Geometry: final body of the model. Coordinates: model frame, mm. A direction names the side the tool comes from. Give positions to 0.01 mm unless a question says otherwise; leave off trailing zeros. Loops run counter-clockwise (first coordinate to the right, second up) from the corner with the lowest first, then second, coordinate; pieces in that order, holes last. Notation, with made-up numbers: M 88,-34.75 L 94,-34.75 A19 cw 94,-22.75 Z; hole C 80,-39 d10. An arc over 180 degrees is marked long. Put each result on its own line as item: value.
```python
from build123d import *

# Parameters (mm, degrees)
SKETCH2_W               = 9.652
SKETCH2_H               = 3.048
SKETCH2_W_2             = 3.048
SKETCH2_H_2             = 35.052
BOSS_EXTRUDE1_DEPTH     = 195
CUT_EXTRUDE1_DEPTH      = 323.7
CUT_EXTRUDE1_DEPTH_BACK = 1


with BuildPart() as part:
    # Sketch2 → Boss-Extrude1 (new body)
    with BuildSketch(Plane.XY):
        Polygon((-12.7, 0), (-9.652, 0), (-9.652, 35.052), (-9.652, 38.1), (-12.7, 38.1), align=None)
        with Locations((-4.826, 36.576)):
            Rectangle(SKETCH2_W, SKETCH2_H)
        Polygon((0, 38.1), (0, 35.052), (9.652, 35.052), (9.652, 0), (12.7, 0), (12.7, 38.1), align=None)
        with Locations((11.176, -17.526)):
            Rectangle(SKETCH2_W_2, SKETCH2_H_2)
        Polygon((-9.652, -35.052), (-9.652, 0), (-12.7, 0), (-12.7, -38.1), (0, -38.1), (0, -35.052), align=None)
        Polygon((9.652, -35.052), (0, -35.052), (0, -38.1), (12.7, -38.1), (12.7, -35.052), align=None)
    extrude(amount=BOSS_EXTRUDE1_DEPTH)

    # Sketch3 → Cut-Extrude1 (cut, two sides)
    with BuildSketch(Plane(origin=(310, 0, 195), x_dir=(0, 0, 1), z_dir=(-1, 0, 0))) as cut_extrude1_sk:
        Polygon((-12.7, -38.1), (-12.7, 38.1), (12.7, 38.1), align=None)
        Polygon((12.7, -38.1), (-12.7, -38.1), (12.7, 38.1), align=None)
        Polygon((-182.3, 38.1), (-207.7, 38.1), (-207.7, -38.1), align=None)
        Polygon((-182.3, -38.1), (-207.7, -38.1), (-182.3, 38.1), align=None)
    extrude(amount=CUT_EXTRUDE1_DEPTH, mode=Mode.SUBTRACT)
    extrude(cut_extrude1_sk.sketch, amount=-CUT_EXTRUDE1_DEPTH_BACK, mode=Mode.SUBTRACT)


solid = part.part
```
Item 1: Section A-A on x = 5.75. Output: boundary loops of the cut face in (y, z).
Output values:
outline: M -38.1,12.7 L -35.05,12.7 L -35.05,182.3 L -38.1,182.3 Z; M 35.05,12.7 L 38.1,12.7 L 38.1,182.3 L 35.05,182.3 Z
Item 2: Mould query, pull axis X, two halves, no side actions, for faces 1 (the flat face through (9.652, 0, 96)), 2 (the flat face through (-10, -3, 182.3)), 3 (the flat face through (0, 35.052, 96)), 4 (the flat face through (12.7, -1, 96)). Classes: pulls with the +X half, pulls with the -X half, needs draft (parallel to the pull), parting line crosses it, or undercut.
Output values:
face 1: undercut
face 2: needs draft
face 3: undercut
face 4: pulls with the +X half
Item 3: Set-up query: faces 5 (the flat face through (-9.652, 0, 96)), 6 (the flat face through (0, -38.1, 96)). Return all of +Z, -Z, +X, -X, +Y, -Y with unobstructed straight access to the full face (end or side cutting, diameter ignored); none if empty.
Output values:
face 5: +Z, -Z
face 6: +Z, -Z, +X, -X, -Y
Item 4: Line query: probe 1 along X at (y, z) = (-25.5, 76.5); probe 2 along Y at (x, z) = (0.5, 26.5). Output: solid intervals per line, ascending. Write a range as [from, to].
Output values:
probe 1: [-12.7, -9.65], [9.65, 12.7]
probe 2: [-38.1, -35.05], [35.05, 38.1]
Item 5: Section B-B on y = 16. Output: boundary loops of the cut face in (x, z), then the cut area to 3 significant figures.
Output values:
outline: M -12.7,12.7 L -9.65,12.7 L -9.65,182.3 L -12.7,182.3 Z; M 9.65,12.7 L 12.7,12.7 L 12.7,182.3 L 9.65,182.3 Z
area: 1,030 mm²
Item 6: Section C-C on z = 145. Output: boundary loops of the cut face in (x, y).
Output values:
outline: M -12.7,-38.1 L 12.7,-38.1 L 12.7,38.1 L -12.7,38.1 Z; hole M -9.65,-35.05 L 9.65,-35.05 L 9.65,35.05 L -9.65,35.05 Z
Item 7: Pin query (flat end, axial travel): pin 1 Ø1.5 at (x, y) = (-7.5, 21.5) entering from +Z. Return the tip coordinate at first contact, or that it passes through.
Output values:
pin 1: through
